Check sheet for the modelled part. Datum: model origin and axes. Units: mm. A direction names the side the tool comes from. Coordinates: 2 decimals unless noted, no trailing zeros. Loops run counter-clockwise (first coordinate to the right, second up) from the corner with the lowest first, then second, coordinate; pieces in that order, holes last. Notation, with made-up numbers: M 33.25,54 L 89.25,54 A27 ccw 89.25,80 Z; hole C -2,21 d11. An arc over 180 degrees is marked long. Return JSON: item names as keys, results as strings.
from build123d import *

# Parameters (mm, degrees)
BASE_EXTRUDE_DEPTH       = 4
SKETCH2_W                = 3.8
SKETCH2_H                = 6
BOSS_EXTRUDE1_DEPTH      = 1
SKETCH3_W                = 3.2
SKETCH3_H                = 5.8
BOSS_EXTRUDE2_DEPTH      = 6
BOSS_EXTRUDE3_DEPTH      = 2.2
WIRE_INSULATION_SKETCH_R = 0.75
WIRE_INSULATION_DEPTH    = 50
WIRE_SKETCH_R            = 0.375
WIRE_2_DEPTH             = 5
CHAMFER1_SIZE            = 0.1


with BuildPart() as part:
    # Sketch1 → Base-Extrude (new body)
    with BuildSketch(Plane(origin=(0, 0, 0), x_dir=(1, 0, 0), z_dir=(0, 1, 0))):
        Polygon((3.9, 3), (3.9, 3.5), (-2.2, 3.5), (-2.2, -3.5), (3.9, -3.5), (3.9, -3), (1.6, -3), (1.6, 3), align=None)
    extrude(amount=BASE_EXTRUDE_DEPTH)

    # Sketch2 → Boss-Extrude1 (add)
    with BuildSketch(Plane(origin=(0, 4, 0), x_dir=(-1, 0, 0), z_dir=(0, 1, 0))):
        with Locations((0.3, 0)):
            Rectangle(SKETCH2_W, SKETCH2_H)
    extrude(amount=BOSS_EXTRUDE1_DEPTH)

    # Sketch3 → Boss-Extrude2 (add)
    with BuildSketch(Plane.XZ):
        Rectangle(SKETCH3_W, SKETCH3_H)
    extrude(amount=BOSS_EXTRUDE2_DEPTH)

    # Sketch4 → Boss-Extrude3 (add, symmetric)
    with BuildSketch(Plane.XY):
        Polygon((1.6, 0), (1.6, 1), (2.9, 1), (2.9, 4), (3.9, 4), (3.9, -3.9), (3.645220836, -4.6), (2.9, -4.6), (2.9, -4.35), (2.5, -4.069916985), (2.5, -3.569916985), (2.9, -3.569916985), (2.9, 0), align=None)
    extrude(amount=BOSS_EXTRUDE3_DEPTH, both=True)

    # Wire Insulation Sketch → Wire Insulation (add)
    with BuildSketch(Plane(origin=(0, 5, 0), x_dir=(-1, 0, 0), z_dir=(0, 1, 0))):
        with Locations(Location((-0.3, 1.25, 0), (0, 0, 90))):
            Circle(WIRE_INSULATION_SKETCH_R)
        with Locations(Location((-0.3, -1.25, 0), (0, 0, 90))):
            Circle(WIRE_INSULATION_SKETCH_R)
    extrude(amount=WIRE_INSULATION_DEPTH)

    # Wire Sketch → Wire 2 (add)
    with BuildSketch(Plane(origin=(0, 55, 0), x_dir=(-1, 0, 0), z_dir=(0, 1, 0))):
        with Locations(Location((-0.3, -1.25, 0), (0, 0, 90))):
            Circle(WIRE_SKETCH_R)
        with Locations(Location((-0.3, 1.25, 0), (0, 0, 90))):
            Circle(WIRE_SKETCH_R)
    extrude(amount=WIRE_2_DEPTH)

    # Chamfer1
    chamfer1_edges = [part.edges().sort_by_distance(p)[0] for p in [
        (0.85, 0, 3.5),
        (-2.2, 0, 0),
        (0.85, 0, -3.5),
    ]]
    chamfer(chamfer1_edges, length=CHAMFER1_SIZE)


solid = part.part
1) Scan lines: line 1 along Y through (x, z) = (-2, 0.5); line 2 along X through (y, z) = (57.5, -1.25) (3 decimals); line 3 along Y through (x, z) = (-0.5, 1). Record each from-to range of solid material in increasing order. Write a range as [from, to].
Answers:
{"line 1": "[0, 5]", "line 2": "[-0.075, 0.675]", "line 3": "[-6, 5]"}
2) Draft check along Z on faces 1 (the face through (2.9, -2, 0)), 2 (the face through (-0.3, 4.5, -3)), 3 (the face through (2, 1, 0)), 4 (the face through (0.81, 29.65, 0.7)). Enter one of: +Z half, -Z half, draft (parallel to the pull), parting line (faces both ways), or undercut.
Answers:
{"face 1": "draft", "face 2": "-Z half", "face 3": "undercut", "face 4": "undercut"}
3) Section check B-B on y = 18. Record the cut outline in (x, z).
Answers:
{"outline": "C 0.3,-1.25 d1.5; C 0.3,1.25 d1.5"}
4) Section check A-A on x = -1. Record the cut outline in (y, z), then the cut area to 3 significant figures.
Answers:
{"outline": "M -6,-2.9 L 0,-2.9 L 0,-3.4 L 0.1,-3.5 L 4,-3.5 L 4,-3 L 5,-3 L 5,3 L 4,3 L 4,3.5 L 0.1,3.5 L 0,3.4 L 0,2.9 L -6,2.9 Z", "area": "68.8 mm²"}
5) Go/stop test with flat-tipped pins: pin 1 Ø0.6 at (x, z) = (2, -3) entering from +Y; pin 2 Ø3 at (x, y) = (2, 12) entering from +Z; pin 3 Ø1 at (x, z) = (2.5, 0) entering from -Y; pin 4 Ø3 at (x, z) = (-0.5, -0.5) entering from +Y. Record where each tip stops, or that it passes through.
Answers:
{"pin 1": "y = 4", "pin 2": "z = 1.97", "pin 3": "y = -4.6", "pin 4": "y = 60"}
6) Set-up check for faces 5 (the face through (0.525, 29.65, -0.535)), 6 (the face through (3.4, 4, 0)), 7 (the face through (3, 2, -3)): record each of +Z, -Z, +X, -X, +Y, -Y from which the full face is reachable in a straight line by a thin tool's end or side.
Answers:
{"face 5": "+Y", "face 6": "+Z, -Z, +X, +Y", "face 7": "+X, +Y, -Y"}
